Autodesk Inventor part; units mm, degrees
ref_plane "YZ Plane" through (0, 0, 0) normal (1, 0, 0) x (0, 1, 0)
ref_plane "XZ Plane" through (0, 0, 0) normal (0, 1, 0) x (-1, 0, 0)
ref_plane "XY Plane" through (0, 0, 0) normal (0, 0, 1) x (1, 0, 0)
sketch "Sketch1" plane through (0, 0, 0) normal (0, 0, 1) x (1, 0, 0)
  line L0 (8, 0) -> (22, 0)
  line L1 (30, 8) -> (30, 47)
  line L2 (27, 50) -> (0, 50)
  line L3 (0, 32.4269) -> (0, 8)
  line L4 (0, 50) -> (0, 35)
  line L5 (30, 50) -> (21.9614, 50)
  line L6 (20.2177, 49.4412) -> (2.0938, 36.4956)
  arc A0 (0, 8) -> (8, 0) centre (8, 8) ccw
  arc A1 (22, 0) -> (30, 8) centre (22, 8) ccw
  arc A2 (30, 47) -> (27, 50) centre (27, 47) ccw
  arc A3 (2.0938, 36.4956) -> (0, 32.4269) centre (5, 32.4269) ccw
  arc A4 (21.9614, 50) -> (20.2177, 49.4412) centre (21.9614, 47) ccw
  point P0 (0, 0)
  point P1 (30, 0)
  point P2 (21, 50)
  dimension "d0" = 30
  dimension "d1" = 50
  dimension "d2" = 15
  dimension "d3" = 9
  dimension "d4" = 8
  dimension "d21" = 3
  dimension "d22" = 5
  dimension "d23" = 3
extrude "Extrusion1" add sketch "Sketch1" along normal blind 10
fillet "Fillet1" radius 1 14 edges at (2.3431, 2.3431, 10) (15, 0, 10) (27.6569, 2.3431, 10) (30, 27.5, 10) (0, 20.2135, 10) (11.1557, 42.9684, 10) (24.4807, 50, 10) (24.4807, 50, 0) (11.1557, 42.9684, 0) (2.3431, 2.3431, 0) (15, 0, 0) (27.6569, 2.3431, 0) (30, 27.5, 0) (0, 20.2135, 0)
sketch "Sketch2" plane through (8, 0, 9) normal (0, -1, 0) x (1, 0, 0)
  line L0 (4.5, -4.925) -> (9.5, -4.925)
  line L1 (9.5, -4.925) -> (9.5, -2.425)
  line L2 (9.5, -2.425) -> (4.5, -2.425)
  line L3 (4.5, -2.425) -> (4.5, -4.925)
  line L4 (22, -8) -> (22, 0)
  line L5 (-8, -8) -> (-8, 0)
  line L6 (0, -9) -> (14, -9)
  line L7 (14, 1) -> (0, 1)
  line L8 (11, -6.425) -> (3, -6.425)
  line L9 (3, -6.425) -> (3, -0.925)
  line L10 (3, -0.925) -> (11, -0.925)
  line L11 (11, -0.925) -> (11, -6.425)
  point P0 (-8, -9)
  dimension "d8" = 5
  dimension "d9" = 2.5
  dimension "d10" = 30
  dimension "d11" = 12.5
  dimension "d12" = 10
  dimension "d13" = 3.425
  dimension "d14" = 1.5
extrude "Extrusion2" add sketch "Sketch2" along normal blind 10
sketch "Sketch3" plane through (11, 0, 8.075) normal (0, 0, 1) x (1, 0, 0)
  circle A0 centre (4.0603, -2.2) radius 0.75
  line L0 (8, -10) -> (0, -10)
  point P0 (-11, 0)
  dimension "d17" = 1.5
  dimension "d18" = 7.8
extrude "Extrusion3" cut sketch "Sketch3" against normal up to surface (5.5 mm away)
Model file for the job. Use its own axes, mm. A direction names the side the tool comes from. Give positions to 0.01 mm unless a question says otherwise; leave off trailing zeros. Write each loop counter-clockwise with the first axis right and the second up, starting at its lowest first coordinate (ties: lowest second). Pieces come first, ordered by that corner, then holes. Notation, with made-up numbers: M 27,28.25 L 55,28.25 A25 cw 55,49.25 Z; hole C 3,61.5 d6. An arc over 180 degrees is marked long. Use a Markdown table: item, result.
1) Cut at A-A (y = -2.2). List the corners of the cut face in (x, z) (3 decimals), and give its area (3 significant figures).
Responses:
| item | result |
|---|---|
| outline | M 11,2.575 L 14.31,2.575 L 14.31,4.075 L 12.5,4.075 L 12.5,6.575 L 14.31,6.575 L 14.31,8.075 L 11,8.075 Z; M 15.81,2.575 L 19,2.575 L 19,8.075 L 15.81,8.075 L 15.81,6.575 L 17.5,6.575 L 17.5,4.075 L 15.81,4.075 Z |
| area | 27.0 mm2 |
2) Pull direction X, two halves, no side cores. Call faces 1 (the cylindrical face through (0.54, 34.69, 4.94)), 2 (the flat face through (15, -5, 4.075)), 3 (the flat face through (15, -5, 2.575)): +X half, -X half, draft (parallel to the pull), parting line (faces both ways), or undercut.
Responses:
| item | result |
|---|---|
| face 1 | -X half |
| face 2 | undercut |
| face 3 | draft |
3) Pin check, flat tips, straight feed: pin 1 (5.5 mm diameter, centred on x = 15, y = -7.5, fed in from +Z) (3 decimals); pin 2 (3 mm diameter, centred on x = 14, z = 5, fed in from -Y); pin 3 (3 mm diameter, centred on y = -5.5, z = 5, fed in from +X); pin 4 (4 mm diameter, centred on x = 14, y = -5.5, fed in from -Z) (3 decimals). Stop position of each tip, or through.
Responses:
| item | result |
|---|---|
| pin 1 | stops at z = 8.075 |
| pin 2 | stops at y = -10 |
| pin 3 | stops at x = 19 |
| pin 4 | stops at z = 2.575 |
4) Cut at B-B (z = 5.25). List the corners of the cut face in (x, y).
Responses:
| item | result |
|---|---|
| outline | M 0,8 A8 ccw 8,0 L 11,0 L 11,-10 L 12.5,-10 L 12.5,0 L 17.5,0 L 17.5,-10 L 19,-10 L 19,0 L 22,0 A8 ccw 30,8 L 30,47 A3 ccw 27,50 L 21.96,50 A3 ccw 20.22,49.44 L 2.09,36.5 A5 ccw 0,32.43 Z |
5) Drill centre lines: line 1 (Y direction, x = 20.75, z = 2); line 2 (Y direction, x = 10, z = 5.5); line 3 (X direction, y = 2.5, z = 1.75). Where is each one in solid material? Low to high. Write a range as from..to.
Responses:
| item | result |
|---|---|
| line 1 | y = 0..49.74 |
| line 2 | y = 0..42.14 |
| line 3 | x = 2.19..27.81 |
6) Tool access for faces 4 (the flat face through (15, 0, 5)), 5 (the cylindrical face through (11.195, 42.646, 0.301)), 6 (the flat face through (19, -5, 5)): list every direction of +Z, -Z, +X, -X, +Y, -Y with a clear straight run to the whole face (end or side of a thin tool).
Responses:
| item | result |
|---|---|
| face 4 | -Y |
| face 5 | -Z, -X, +Y |
| face 6 | +Z, -Z, +X, -Y |
